```python
from build123d import *

# Parameters (mm, degrees)
ESQUISSE1_W             = 10
ESQUISSE1_H             = 8
ESQUISSE1_W_2           = 30
ESQUISSE1_H_2           = 1.2
BOSS_EXTRU_1_DEPTH      = 33
ENL_V_MAT_EXTRU_3_DEPTH = 30
BOSS_EXTRU_2_DEPTH      = 2
ESQUISSE4_R             = 1.5
ENL_V_MAT_EXTRU_4_DEPTH = 10
ENL_V_MAT_EXTRU_5_DEPTH = 53.469038489


with BuildPart() as part:
    # Esquisse1 → Boss.-Extru.1 (new body)
    with BuildSketch(Plane.XY):
        with Locations((-35, 4)):
            Rectangle(ESQUISSE1_W, ESQUISSE1_H)
        with Locations((5, 4)):
            Rectangle(ESQUISSE1_W, ESQUISSE1_H)
        with Locations((-15, 0.6)):
            Rectangle(ESQUISSE1_W_2, ESQUISSE1_H_2)
    extrude(amount=BOSS_EXTRU_1_DEPTH)

    # Esquisse2 → Enlèv. mat.-Extru.3 (cut)
    with BuildSketch(Plane.XZ):
        with BuildLine():
            Line((-4.5, 0), (-4.5, 12))
            ThreePointArc((-4.5, 12), (-15, 22.5), (-25.5, 12))
            Line((-25.5, 12), (-25.5, 0))
            Line((-25.5, 0), (-4.5, 0))
        make_face()
    extrude(amount=-ENL_V_MAT_EXTRU_3_DEPTH, mode=Mode.SUBTRACT)

    # Esquisse3 → Boss.-Extru.2 (add)
    with BuildSketch(Plane(origin=(0, 1.2, 0), x_dir=(1, 0, 0), z_dir=(0, 1, 0))):
        with BuildLine():
            ThreePointArc((-1, -12), (-15, -26), (-29, -12))
            Line((-29, -12), (-29, 0))
            Line((-29, 0), (-30, 0))
            Line((-30, 0), (-30, -33))
            Line((-30, -33), (0, -33))
            Line((0, -33), (0, 0))
            Line((0, 0), (-1, 0))
            Line((-1, 0), (-1, -12))
        make_face()
    extrude(amount=BOSS_EXTRU_2_DEPTH)

    # Esquisse4 → Enlèv. mat.-Extru.4 (cut)
    with BuildSketch(Plane(origin=(0, 0, 0), x_dir=(-1, 0, 0), z_dir=(0, 0, -1))):
        with Locations((35, 4)):
            Circle(ESQUISSE4_R)
        with Locations((-5, 4)):
            Circle(ESQUISSE4_R)
    extrude(amount=-ENL_V_MAT_EXTRU_4_DEPTH, mode=Mode.SUBTRACT)

    # Esquisse5 → Enlèv. mat.-Extru.5 (cut, through all)
    with BuildSketch(Plane.XZ):
        with BuildLine():
            Line((-40, 33), (-40, 16.5))
            ThreePointArc((-40, 16.5), (-29.977065819, 28.503129989), (-15.000000044, 33))
            Line((-15.000000044, 33), (-40, 33))
        make_face()
        with BuildLine():
            Line((10, 33), (-15.000000044, 33))
            ThreePointArc((-15.000000044, 33), (-0.022934218, 28.503130013), (10, 16.5))
            Line((10, 16.5), (10, 33))
        make_face()
    extrude(amount=-ENL_V_MAT_EXTRU_5_DEPTH, mode=Mode.SUBTRACT)


solid = part.part
```
Input: part model. Units: mm. Frame: model coordinates. A direction names the side the tool comes from. Round coordinates to 2 decimals unless told otherwise and drop trailing zeros. Write each loop counter-clockwise with the first axis right and the second up, starting at its lowest first coordinate (ties: lowest second). Pieces come first, ordered by that corner, then holes. Notation, with made-up numbers: M 66,-31 L 122,-31 A19 ccw 122,-10 Z; hole C 48,89 d4. An arc over 180 degrees is marked long. Write each question's results on one line, items separated by ' | '.
Q1. Section query B-B (z = 11.5). Return loops of the section in (x, y).
Results:
outline: M -40,0 L -25.5,0 L -25.5,1.2 L -29,1.2 L -29,3.2 L -30,3.2 L -30,8 L -40,8 Z; M -4.5,0 L 10,0 L 10,8 L 0,8 L 0,3.2 L -1,3.2 L -1,1.2 L -4.5,1.2 Z
Q2. Line query: line 1 along X through (y, z) = (7.75, 7); line 2 along X through (y, z) = (3, 6); line 3 along Y through (x, z) = (5, 6.5). Output: solid intervals per line, ascending.
Results:
line 1: x = -40 to -30, 0 to 10 | line 2: x = -40 to -36.12, -33.88 to -29, -1 to 3.88, 6.12 to 10 | line 3: y = 0 to 2.5, 5.5 to 8
Q3. Section query C-C (x = -35). Return loops of the section in (y, z), and give its area (3 significant figures).
Results:
outline: M 0,0 L 2.5,0 L 2.5,10 L 5.5,10 L 5.5,0 L 8,0 L 8,24.23 L 0,24.23 Z | area: 164 mm^2
Q4. Section query A-A (y = 6). Return loops of the section in (x, z).
Results:
outline: M -40,0 L -30,0 L -30,28.49 A27.19 ccw -40,16.5 Z; M 0,0 L 10,0 L 10,16.5 A27.19 ccw 0,28.49 Z
Q5. Section query D-D (x = 2.5). Return loops of the section in (y, z), and give its area (3 significant figures).
Results:
outline: M 0,0 L 8,0 L 8,26.62 L 0,26.62 Z | area: 213 mm^2
Q6. Access query for faces 4 (the face through (-25.5, 1, 6)), 5 (the face through (-1, 2, 6)), 6 (the face through (-30, 6, 14)), 7 (the face through (-33.8, 3.1, 4.9)). Directions: +Z, -Z, +X, -X, +Y, -Y. A direction counts if a zero-diameter tool reaches every point of the face in a straight line with its end or side. Return the directions, or none.
Results:
face 4: -Z, +Y, -Y | face 5: -Z, +Y | face 6: +Z, -Z, +Y | face 7: -Z
Q7. Pin query (flat end, axial travel): P1, Ø4, axis at y = 7, z = 21, coming from the +X side; P2, Ø2.5, axis at x = -35, y = 4, coming from the -Z side; P3, Ø3, axis at y = 2, z = 23, coming from the +X side; P4, Ø3, axis at x = -19.5, y = 5, coming from the -Z side. Return the tip coordinate at first contact, or that it passes through.
Results:
P1: stops at x = 8.78 | P2: stops at z = 10 | P3: stops at x = 7.21 | P4: passes through
Q8. Draft query along X for faces 1 (the face through (-15.1, 3.2, 26.2)), 2 (the face through (-34, 2, 0)), 3 (the face through (-40, 4, 8)). Return one class per face: released by +X, released by -X, zero draft, split by the parting line, or undercut.
Results:
face 1: undercut | face 2: zero draft | face 3: released by -X
